```python
from build123d import *

# Parameters (mm, degrees)
F0_R     = 2.75
F1_DEPTH = 1.9
F2_R     = 1.5
F3_DEPTH = 23.1
F5_START = 0.5
F5_DEPTH = 4.5
F6_SIZE2 = 1.24999
F6_SIZE  = 1.24999


# Not quite as in the source:
# - a fillet or chamfer is up to 0.001 mm smaller than in the source, because OpenCascade refuses the exact size


with BuildPart() as f1:
    # F0 (on Front) → F1 (new body)
    with BuildSketch(Plane.XZ):
        Circle(F0_R)
    extrude(amount=F1_DEPTH)

    # F2 (on face) → F3 (join)
    with BuildSketch(Plane(origin=(0, 0, 0), x_dir=(-1, 0, 0), z_dir=(0, 1, 0))):
        Circle(F2_R)
    extrude(amount=F3_DEPTH)

    # F4 (on Front) → F5 (cut)
    with BuildSketch(Plane.XZ.offset(F5_START)):
        Polygon((1.1547005384, 0), (0.5773502692, 1), (-0.5773502692, 1), (-1.1547005384, 0), (-0.5773502692, -1), (0.5773502692, -1), align=None)
    extrude(amount=F5_DEPTH, mode=Mode.SUBTRACT)

    # F6 (size 1.25 and 1.25 in the source; OpenCascade refuses exactly that, so slightly less here)
    f6_edges = [f1.edges().sort_by_distance(p)[0] for p in [
        (-2.75, 0, 0),
    ]]
    chamfer(f6_edges, length=F6_SIZE, length2=F6_SIZE2)


solid = f1.part
```
Here's how the part is built. I have some questions about the finished solid (model axes, mm). A direction names the side the tool comes from. Round coordinates to 2 decimals unless told otherwise and drop trailing zeros. Loops run counter-clockwise (first coordinate to the right, second up) from the corner with the lowest first, then second, coordinate; pieces in that order, holes last. Notation, with made-up numbers: (22, -27) -> (62, -27) arc R27 ccw to (62, 6) -> close; hole circle Ø1 at (48, 27). An arc over 180 degrees is marked (long way). Answer as CSV lines item,"result". Start each with the question number.
1. If we mould it in two halves opening along X, with no side actions, what happens to faces 1 (the face through (0.87, -1.19, 0.49)), 2 (the face through (0, -1.9, -1.2)), 3 (the face through (1.5, 11.39, 0.07))? For each: pulls with the +X half, pulls with the -X half, needs draft (parallel to the pull), parting line crosses it, or undercut.
2. I'm going to push flat-ended pins straight in: P1, Ø3, axis at y = 11.5, z = 0.5, coming from the -X side; P2, Ø3, axis at x = -1, y = 6.5, coming from the +Z side; P3, Ø1, axis at x = -1, y = 20.5, coming from the -Z side; P4, Ø0.9, axis at x = 0, y = -1, coming from the +Z side. Where does each tip first touch, or does it pass through?
3. I need wall thicknesses on probe 1 along Y at (x, z) = (-0.4, 0.2); probe 2 along Z at (x, y) = (-0.95, 9.75); probe 3 along X at (y, z) = (19.75, -0.3). Which ranges of each line are inside material? Lowest first, please. Write a range as from..to.
4. For faces 4 (the face through (-0.86, -1.19, 0.51)), 5 (the face through (0, 23.1, 0)), which set-ups out of +Z, -Z, +X, -X, +Y, -Y let a thin tool reach every point of the face, with its end or its side?
5. Imagine slicing it at B-B on y = 14.5. Write out the boundary of the cut face in (x, z).
Solution:
1,face 1,"undercut"
1,face 2,"needs draft"
1,face 3,"parting line crosses it"
2,P1,"x = -1.5"
2,P2,"z = 1.5"
2,P3,"z = -1.41"
2,P4,"z = 2.75"
3,probe 1,"-0.5..23.1"
3,probe 2,"-1.16..1.16"
3,probe 3,"-1.47..1.47"
4,face 4,"-Y"
4,face 5,"+Z, -Z, +X, -X, +Y"
5,outline,"circle Ø3 at (0, 0)"
